Can you work these out from the model? Positions are in its coordinate system, mm. Face numbers are marked on the shaded views. Give positions to 0.01 mm unless a question says otherwise; leave off trailing zeros. Loops run counter-clockwise (first coordinate to the right, second up) from the corner with the lowest first, then second, coordinate; pieces in that order, holes last. Notation, with made-up numbers: (35.25, -23.5) -> (65.25, -23.5) arc R18 cw to (65.25, -12.5) -> close; hole circle Ø7 at (51.5, -3). An arc over 180 degrees is marked (long way). Use CSV: the item, a comma, the result in double quotes.
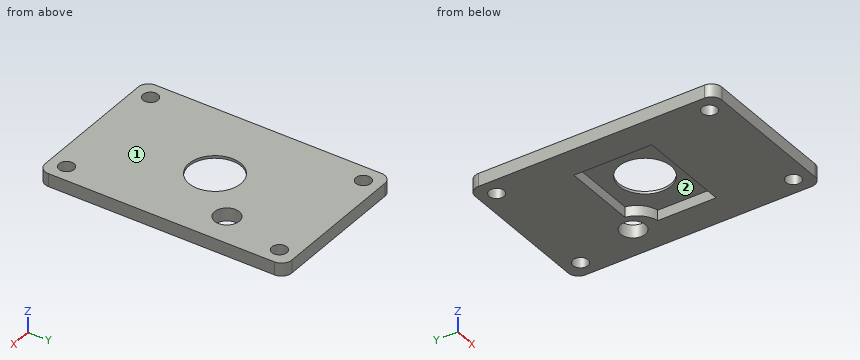
from build123d import *

# Parameters (mm, degrees)
F0_W     = 76.2
F0_H     = 120.65
F0_R     = 3.683
F0_R_2   = 12.7
F0_R_3   = 6.0579
F1_DEPTH = 6.35
F2_R     = 5.08
F3_R     = 12.7
F4_DEPTH = 5.08


# Not quite as in the source:
# - a length typed as a fraction of an inch, garbled in the dataset ("3 / 203.2 mm" for 3/8 in), is restored


with BuildPart() as f1:
    # F0 (on Top) → F1 (new body)
    with BuildSketch(Plane.XY):
        Rectangle(F0_W, F0_H)
        with Locations((-29.8323, -52.0573)):
            Circle(F0_R, mode=Mode.SUBTRACT)
        with Locations((29.8323, -52.0573)):
            Circle(F0_R, mode=Mode.SUBTRACT)
        with Locations((-29.8323, 52.0573)):
            Circle(F0_R, mode=Mode.SUBTRACT)
        Circle(F0_R_2, mode=Mode.SUBTRACT)
        with Locations((22.3901, 21.2471)):
            Circle(F0_R_3, mode=Mode.SUBTRACT)
        with Locations((29.8323, 52.0573)):
            Circle(F0_R, mode=Mode.SUBTRACT)
    extrude(amount=F1_DEPTH)

    # F2
    f2_edges = [f1.edges().sort_by_distance(p)[0] for p in [
        (38.1, -60.325, 3.175),
        (-38.1, 60.325, 3.175),
        (38.1, 60.325, 3.175),
        (-38.1, -60.325, 3.175),
    ]]
    fillet(f2_edges, radius=F2_R)

    # F3 (on face) → F4 (cut)
    with BuildSketch(Plane(origin=(0, 0, 0), x_dir=(1, 0, 0), z_dir=(0, 0, -1))):
        with BuildLine():
            Line((22.86, 19.05), (14.4386043259, 19.05))
            Line((14.4386043259, 19.05), (-22.86, 19.05))
            Line((-22.86, 19.05), (-22.86, -19.05))
            Line((-22.86, -19.05), (13.4802116102, -19.05))
            ThreePointArc((13.4802116102, -19.05), (16.6474146742, -12.7797644882), (22.86, -9.5009213703))
            Line((22.86, -9.5009213703), (22.86, 19.05))
        make_face()
        Circle(F3_R, mode=Mode.SUBTRACT)
    extrude(amount=-F4_DEPTH, mode=Mode.SUBTRACT)


solid = f1.part
(1) If we section it at C-C, the plane z = 3.25: Write out the boundary of the cut face in (x, y) (3 decimals), then the cut area to 3 significant figures.
Answer sheet:
outline,"(-38.1, -55.245) arc R5.08 ccw to (-33.02, -60.325) -> (33.02, -60.325) arc R5.08 ccw to (38.1, -55.245) -> (38.1, 55.245) arc R5.08 ccw to (33.02, 60.325) -> (-33.02, 60.325) arc R5.08 ccw to (-38.1, 55.245) -> close; hole circle Ø7.366 at (-29.832, -52.057); hole circle Ø7.366 at (-29.832, 52.057); hole (-22.86, -19.05) -> (22.86, -19.05) -> (22.86, 9.501) arc R11.56 cw to (13.48, 19.05) -> (-22.86, 19.05) -> close; hole circle Ø12.116 at (22.39, 21.247); hole circle Ø7.366 at (29.832, -52.057); hole circle Ø7.366 at (29.832, 52.057)"
area,"7,210 mm2"
(2) Will these pins go through, and if not, where does the flat tip stop? pin 1 Ø11.5 at (x, y) = (2, -8.5) entering from -Z; pin 2 Ø9.5 at (x, y) = (22.39, 21.25) entering from -Z.
Answer sheet:
pin 1,"stops at z = 5.08"
pin 2,"passes through"
(3) If we section it at B-B, the plane x = 0: Write out the boundary of the cut face in (y, z) (3 decimals), then the cut area to 3 significant figures.
Answer sheet:
outline,"(-60.325, 0) -> (-19.05, 0) -> (-19.05, 5.08) -> (-12.7, 5.08) -> (-12.7, 6.35) -> (-60.325, 6.35) -> close; (12.7, 5.08) -> (19.05, 5.08) -> (19.05, 0) -> (60.325, 0) -> (60.325, 6.35) -> (12.7, 6.35) -> close"
area,"540 mm2"
(4) If we section it at D-D, the plane x = -16.5: Write out the boundary of the cut face in (y, z) (3 decimals).
Answer sheet:
outline,"(-60.325, 0) -> (-19.05, 0) -> (-19.05, 5.08) -> (19.05, 5.08) -> (19.05, 0) -> (60.325, 0) -> (60.325, 6.35) -> (-60.325, 6.35) -> close"
(5) If we section it at A-A, the plane y = 0: Write out the boundary of the cut face in (x, z), then the cut area to 3 significant figures.
Answer sheet:
outline,"(-38.1, 0) -> (-22.86, 0) -> (-22.86, 5.08) -> (-12.7, 5.08) -> (-12.7, 6.35) -> (-38.1, 6.35) -> close; (12.7, 5.08) -> (22.86, 5.08) -> (22.86, 0) -> (38.1, 0) -> (38.1, 6.35) -> (12.7, 6.35) -> close"
area,"219 mm2"
(6) We'd pull the mould along X, two halves only. Please class the marked faces 1 and 2: released by +X, released by -X, zero draft, split by the parting line, or undercut.
Answer sheet:
face 1,"zero draft"
face 2,"undercut"
(7) If I drill on L1, parallel to Y at x = -14, z = 0.5 (3 decimals); L2, parallel to Y at x = 0, z = 6 (3 decimals); L3, parallel to Y at x = -30, z = 2.75 (3 decimals), over which ranges is the centre line in solid material (lowest first)? Write a range as from..to.
Answer sheet:
L1,"y = -60.325..-19.05, 19.05..60.325"
L2,"y = -60.325..-12.7, 12.7..60.325"
L3,"y = -60.325..-55.736, -48.378..48.378, 55.736..60.325"
